from build123d import *

# Parameters (mm, degrees)
BOSS_EXTRU_1_DEPTH      = 15
ESQUISSE6_W             = 100
ESQUISSE6_H             = 15
ENL_V_MAT_EXTRU_1_DEPTH = 200
ENL_V_MAT_EXTRU_2_REACH = 393.106
ESQUISSE7_W             = 80
ESQUISSE7_H             = 70
ENL_V_MAT_EXTRU_4_REACH = 393.106
ESQUISSE8_R             = 2


with BuildPart() as part:
    # Esquisse1 → Boss.-Extru.1 (new body)
    with BuildSketch(Plane(origin=(0, 0, 0), x_dir=(1, 0, 0), z_dir=(0, 1, 0))):
        Polygon((-76.643189126, -51.401333399), (63.356810874, 43.598666601), (163.356810874, 43.598666601), (303.356810874, -51.401333399), (303.356810874, -151.401333399), (163.356810874, -246.401333399), (63.356810874, -246.401333399), (-76.643189126, -151.401333399), align=None)
    extrude(amount=BOSS_EXTRU_1_DEPTH)

    # Esquisse6 → Enlèv. mat.-Extru.1 (cut)
    with BuildSketch(Plane.XY.offset(246.401333399)):
        with Locations((113.356810874, 7.5)):
            Rectangle(ESQUISSE6_W, ESQUISSE6_H)
    extrude(amount=-ENL_V_MAT_EXTRU_1_DEPTH, mode=Mode.SUBTRACT)

    # Esquisse7 → Enlèv. mat.-Extru.2 (cut, up to next)
    with BuildSketch(Plane(origin=(0, 15, 0), x_dir=(1, 0, 0), z_dir=(0, 1, 0)), mode=Mode.PRIVATE) as enl_v_mat_extru_2_sk1:
        with Locations((-16.643189126, -101.401333399)):
            Rectangle(ESQUISSE7_W, ESQUISSE7_H)
    enl_v_mat_extru_2_tool1 = extrude(enl_v_mat_extru_2_sk1.sketch, amount=-ENL_V_MAT_EXTRU_2_REACH, mode=Mode.PRIVATE) & part.part
    # Esquisse7 → Enlèv. mat.-Extru.2 (cut, up to next)
    with BuildSketch(Plane(origin=(0, 15, 0), x_dir=(1, 0, 0), z_dir=(0, 1, 0)), mode=Mode.PRIVATE) as enl_v_mat_extru_2_sk2:
        with Locations((243.356810874, -101.401333399)):
            Rectangle(ESQUISSE7_W, ESQUISSE7_H)
    enl_v_mat_extru_2_tool2 = extrude(enl_v_mat_extru_2_sk2.sketch, amount=-ENL_V_MAT_EXTRU_2_REACH, mode=Mode.PRIVATE) & part.part
    add(enl_v_mat_extru_2_tool1.solids().sort_by_distance((-16.643189, 15, 101.401333))[0], mode=Mode.SUBTRACT)
    add(enl_v_mat_extru_2_tool2.solids().sort_by_distance((243.356811, 15, 101.401333))[0], mode=Mode.SUBTRACT)

    # Esquisse8 → Enlèv. mat.-Extru.4 (cut, up to next)
    with BuildSketch(Plane(origin=(0, 15, 0), x_dir=(1, 0, 0), z_dir=(0, 1, 0)), mode=Mode.PRIVATE) as enl_v_mat_extru_4_sk1:
        with Locations(Location((180.356810874, -120.901333399, 0), (0, 0, 270))):
            Circle(ESQUISSE8_R)
    enl_v_mat_extru_4_tool1 = extrude(enl_v_mat_extru_4_sk1.sketch, amount=-ENL_V_MAT_EXTRU_4_REACH, mode=Mode.PRIVATE) & part.part
    # Esquisse8 → Enlèv. mat.-Extru.4 (cut, up to next)
    with BuildSketch(Plane(origin=(0, 15, 0), x_dir=(1, 0, 0), z_dir=(0, 1, 0)), mode=Mode.PRIVATE) as enl_v_mat_extru_4_sk2:
        with Locations(Location((180.356810874, -81.901333399, 0), (0, 0, 270))):
            Circle(ESQUISSE8_R)
    enl_v_mat_extru_4_tool2 = extrude(enl_v_mat_extru_4_sk2.sketch, amount=-ENL_V_MAT_EXTRU_4_REACH, mode=Mode.PRIVATE) & part.part
    # Esquisse8 → Enlèv. mat.-Extru.4 (cut, up to next)
    with BuildSketch(Plane(origin=(0, 15, 0), x_dir=(1, 0, 0), z_dir=(0, 1, 0)), mode=Mode.PRIVATE) as enl_v_mat_extru_4_sk3:
        with Locations(Location((46.356810874, -120.901333399, 0), (0, 0, 270))):
            Circle(ESQUISSE8_R)
    enl_v_mat_extru_4_tool3 = extrude(enl_v_mat_extru_4_sk3.sketch, amount=-ENL_V_MAT_EXTRU_4_REACH, mode=Mode.PRIVATE) & part.part
    # Esquisse8 → Enlèv. mat.-Extru.4 (cut, up to next)
    with BuildSketch(Plane(origin=(0, 15, 0), x_dir=(1, 0, 0), z_dir=(0, 1, 0)), mode=Mode.PRIVATE) as enl_v_mat_extru_4_sk4:
        with Locations(Location((46.356810874, -81.901333399, 0), (0, 0, 270))):
            Circle(ESQUISSE8_R)
    enl_v_mat_extru_4_tool4 = extrude(enl_v_mat_extru_4_sk4.sketch, amount=-ENL_V_MAT_EXTRU_4_REACH, mode=Mode.PRIVATE) & part.part
    add(enl_v_mat_extru_4_tool1.solids().sort_by_distance((180.356811, 15, 120.901333))[0], mode=Mode.SUBTRACT)
    add(enl_v_mat_extru_4_tool2.solids().sort_by_distance((180.356811, 15, 81.901333))[0], mode=Mode.SUBTRACT)
    add(enl_v_mat_extru_4_tool3.solids().sort_by_distance((46.356811, 15, 120.901333))[0], mode=Mode.SUBTRACT)
    add(enl_v_mat_extru_4_tool4.solids().sort_by_distance((46.356811, 15, 81.901333))[0], mode=Mode.SUBTRACT)


solid = part.part
Check sheet for the modelled part. Datum: model origin and axes. Units: mm. A direction names the side the tool comes from. Give positions to 0.01 mm unless a question says otherwise; leave off trailing zeros. Write each loop counter-clockwise with the first axis right and the second up, starting at its lowest first coordinate (ties: lowest second). Pieces come first, ordered by that corner, then holes. Notation, with made-up numbers: (0.25, 18.25) -> (52.25, 18.25) arc R23 ccw to (52.25, 33.25) -> close; hole circle Ø7 at (-37, -21). An arc over 180 degrees is marked (long way). Use one line per item in the form item = value. Start each with the question number.
1. Thickness scan on line 1 along X through (y, z) = (10.75, 125); line 2 along X through (y, z) = (5.5, 148); line 3 along Z through (x, y) = (-27, 13.25). Record the ranges inside material, lowest first. Write a range as from..to.
2. Section check D-D (x = -44). Record the cut outline in (y, z), and give its area (3 significant figures).
3. Section check C-C (y = 11.5). Record the cut outline in (x, z).
4. Mould release check, pull along X, two halves, no side actions. Record for faces 1 (the flat face through (232.38, 7.4, 3.24)), 2 (the flat face through (-17, 8, 66.401)), 3 (the flat face through (-7.623, 7.395, 4.566)): pulls with the +X half, pulls with the -X half, needs draft (parallel to the pull), parting line crosses it, or undercut.
5. Go/stop test with flat-tipped pins: P1, Ø1, axis at x = -28, y = 9, coming from the +Z side; P2, Ø2, axis at x = 229.5, y = 3.5, coming from the +Z side; P3, Ø6, axis at x = 33, y = 5.5, coming from the -Z side. Record where each tip stops, or that it passes through.
6. Section check B-B (z = 103.5). Record the cut outline in (x, y), and give its area (3 significant figures).
7. Access from +Z, -Z, +X, -X, +Y, -Y to the whole of each face (thin tool, end or side, straight path). Record for faces 4 (the flat face through (63.357, 7, 148)), 5 (the flat face through (203.357, 8, 102)), 6 (the flat face through (-76.643, 7, 102)).
8. Section check A-A (z = 143.5). Record the cut outline in (x, y).
Conclusion:
q1.line_1 = -76.64..-56.64, 23.36..63.36, 163.36..203.36, 283.36..303.36
q1.line_2 = -76.64..63.36, 163.36..303.36
q1.line_3 = 17.71..66.4, 136.4..185.09
q2.outline = (0, 29.25) -> (15, 29.25) -> (15, 66.4) -> (0, 66.4) -> close; (0, 136.4) -> (15, 136.4) -> (15, 173.55) -> (0, 173.55) -> close
q2.area = 1,110 mm²
q3.outline = (-76.64, 51.4) -> (63.36, -43.6) -> (163.36, -43.6) -> (303.36, 51.4) -> (303.36, 151.4) -> (163.36, 246.4) -> (163.36, 46.4) -> (63.36, 46.4) -> (63.36, 246.4) -> (-76.64, 151.4) -> close; hole (-56.64, 66.4) -> (23.36, 66.4) -> (23.36, 136.4) -> (-56.64, 136.4) -> close; hole circle Ø4 at (46.36, 81.9); hole circle Ø4 at (46.36, 120.9); hole circle Ø4 at (180.36, 81.9); hole circle Ø4 at (180.36, 120.9); hole (203.36, 66.4) -> (283.36, 66.4) -> (283.36, 136.4) -> (203.36, 136.4) -> close
q4.face_1 = pulls with the +X half
q4.face_2 = undercut
q4.face_3 = pulls with the -X half
q5.P1 = 184.75
q5.P2 = 202.2
q5.P3 = -25.04
q6.outline = (-76.64, 0) -> (-56.64, 0) -> (-56.64, 15) -> (-76.64, 15) -> close; (23.36, 0) -> (63.36, 0) -> (63.36, 15) -> (23.36, 15) -> close; (163.36, 0) -> (203.36, 0) -> (203.36, 15) -> (163.36, 15) -> close; (283.36, 0) -> (303.36, 0) -> (303.36, 15) -> (283.36, 15) -> close
q6.area = 1,800 mm²
q7.face_4 = +Z, +Y, -Y
q7.face_5 = +Y, -Y
q7.face_6 = +Z, -Z, -X, +Y, -Y
q8.outline = (-76.64, 0) -> (63.36, 0) -> (63.36, 15) -> (-76.64, 15) -> close; (163.36, 0) -> (303.36, 0) -> (303.36, 15) -> (163.36, 15) -> close
